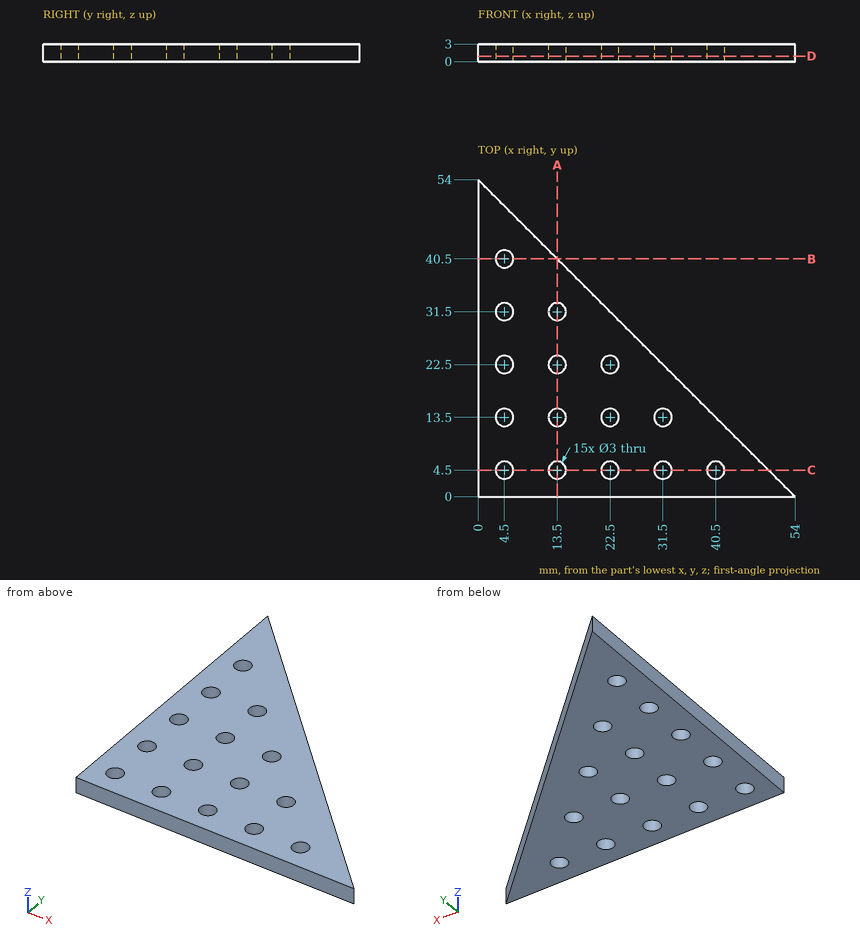
Part print with two shaded views. Sizes in mm from the minimum x, y, z corner. Round coordinates to 2 decimals unless told otherwise and drop trailing zeros. Loops run counter-clockwise (first coordinate to the right, second up) from the corner with the lowest first, then second, coordinate; pieces in that order, holes last. Notation, with made-up numbers: M 59,10 L 83,10 A22 cw 83,32 Z; hole C 81,64.5 d4. An arc over 180 degrees is marked long. Put each result on its own line as item: value. Start each with the question number.
Item 1: Cut at D-D (z = 0.95). Give the number of separate pieces and of enclosed holes in the cut face, then the cut area to 3 significant figures.
Item 2: Drop a flat-ended pin along its axis: P1, Ø1.8, axis at x = 31.5, y = 13.5, coming from the -Z side. Give the stop position or say it passes through.
Item 3: Cut at A-A (x = 13.5). List the corners of the cut face in (y, z).
Item 4: Drill centre lines: line 1 along Y through (x, z) = (22.5, 1.7); line 2 along Y through (x, z) = (4.5, 2.1); line 3 along Y through (x, z) = (14, 0.3). Where is each one in solid material? Low to high.
Item 5: Cut at B-B (y = 40.5). List the corners of the cut face in (x, z).
Item 6: Cut at C-C (y = 4.5). List the corners of the cut face in (x, z), then the cut area to 4 significant figures.
Answer block:
1. separate pieces: 1
1. enclosed holes: 15
1. area: 1,350 mm2
2. P1: through
3. outline: M 0,0 L 3,0 L 3,3 L 0,3 Z; M 6,0 L 12,0 L 12,3 L 6,3 Z; M 15,0 L 21,0 L 21,3 L 15,3 Z; M 24,0 L 30,0 L 30,3 L 24,3 Z; M 33,0 L 40.5,0 L 40.5,3 L 33,3 Z
4. line 1: 0 to 3, 6 to 12, 15 to 21, 24 to 31.5
4. line 2: 0 to 3, 6 to 12, 15 to 21, 24 to 30, 33 to 39, 42 to 49.5
4. line 3: 0 to 3.09, 5.91 to 12.09, 14.91 to 21.09, 23.91 to 30.09, 32.91 to 40
5. outline: M 0,0 L 3,0 L 3,3 L 0,3 Z; M 6,0 L 13.5,0 L 13.5,3 L 6,3 Z
6. outline: M 0,0 L 3,0 L 3,3 L 0,3 Z; M 6,0 L 12,0 L 12,3 L 6,3 Z; M 15,0 L 21,0 L 21,3 L 15,3 Z; M 24,0 L 30,0 L 30,3 L 24,3 Z; M 33,0 L 39,0 L 39,3 L 33,3 Z; M 42,0 L 49.5,0 L 49.5,3 L 42,3 Z
6. area: 103.5 mm2
